Here's how the part is built. I have some questions about the finished solid (model axes, mm). A direction names the side the tool comes from. Round coordinates to 2 decimals unless told otherwise and drop trailing zeros. Write each loop counter-clockwise with the first axis right and the second up, starting at its lowest first coordinate (ties: lowest second). Pieces come first, ordered by that corner, then holes. Notation, with made-up numbers: (-38, -22.75) -> (0, -22.75) arc R20 cw to (0, -11.75) -> close; hole circle Ø8 at (45.5, 75.5). An arc over 180 degrees is marked (long way). Answer in a Markdown table with one row per item. Add a question column.
from build123d import *

# Parameters (mm, degrees)
BASE_EXTRUSION_DEPTH = 6
ESQUISSE2_W          = 2
ESQUISSE2_H          = 4.614800239
BOSS_EXTRU_1_DEPTH   = 1


with BuildPart() as part:
    # Esquisse1 → Base-Extrusion (new body)
    with BuildSketch(Plane.XY):
        with BuildLine():
            Line((-1.429070273, 4.791425482), (-1.172025132, 4.085199761))
            ThreePointArc((-1.172025132, 4.085199761), (0, 4.25), (1.172025132, 4.085199761))
            Line((1.172025132, 4.085199761), (1.429070273, 4.791425482))
            ThreePointArc((1.429070273, 4.791425482), (0, 5), (-1.429070273, 4.791425482))
        make_face()
    extrude(amount=BASE_EXTRUSION_DEPTH)

    # Esquisse2 → Boss.-Extru.1 (add)
    with BuildSketch(Plane.XY.offset(6)):
        with Locations((0, 6.69259988)):
            Rectangle(ESQUISSE2_W, ESQUISSE2_H)
    extrude(amount=BOSS_EXTRU_1_DEPTH)


solid = part.part
Item 1: For P1, Ø1.1, axis at y = 5.5, z = 6.5, coming from the -X side; P2, Ø0.5, axis at y = 7, z = 6.5, coming from the +X side; P3, Ø1.6, axis at x = -0.5, y = 7.5, coming from the -Z side, each with a flat end and sliding along its axis, tell me the tip position at first contact or that it passes through.
Item 2: If we section it at B-B on x = 0.55: Please give me the cut outline in (y, z).
Item 3: I need wall thicknesses on line 1 along X through (y, z) = (5.45, 6.5); line 2 along Z through (x, y) = (0.5, 5.5); line 3 along Y through (x, z) = (0.05, 6.25). Which ranges of each line are inside material? Lowest first, please. Write a range as from..to.
Item 4: If we section it at C-C on z = 6.75: Please give me the cut outline in (x, y), then the cut area to 3 significant figures.
Item 5: If we mould it in two halves opening along X, with no side actions, what happens to faces 1 (the flat face through (1, 6.7, 6.5)), 2 (the flat face through (0, 4.385, 6.5)), 3 (the cylindrical face through (-0.02, 4.25, 2.96))? For each: pulls with the +X half, pulls with the -X half, needs draft (parallel to the pull), parting line crosses it, or undercut.
Item 6: If we section it at D-D on x = -0.15: Please give me the cut outline in (y, z), then the cut area to 3 significant figures.
Item 7: If we section it at A-A on y = 6.65: Please give me the cut outline in (x, z), then the cut area to 3 significant figures.
Item 8: On a 3-axis mill with a long thin cutter (end or side, diameter ignored), from which of +Z, -Z, +X, -X, +Y, -Y can I reach the whole of each face in a straight line? I mean faces 4 (the flat face through (0, 7, 7)), 5 (the cylindrical face through (0, 5, 3)). Say none if no direction works.
Results list:
| question | item | result |
|---|---|---|
| 1 | P1 | x = -1 |
| 1 | P2 | x = 1 |
| 1 | P3 | z = 6 |
| 2 | outline | (4.21, 0) -> (4.97, 0) -> (4.97, 6) -> (9, 6) -> (9, 7) -> (4.39, 7) -> (4.39, 6) -> (4.21, 6) -> close |
| 3 | line 1 | -1..1 |
| 3 | line 2 | 6..7 |
| 3 | line 3 | 4.39..9 |
| 4 | outline | (-1, 4.39) -> (1, 4.39) -> (1, 9) -> (-1, 9) -> close |
| 4 | area | 9.23 mm² |
| 5 | face 1 | pulls with the +X half |
| 5 | face 2 | needs draft |
| 5 | face 3 | undercut |
| 6 | outline | (4.25, 0) -> (5, 0) -> (5, 6) -> (9, 6) -> (9, 7) -> (4.39, 7) -> (4.39, 6) -> (4.25, 6) -> close |
| 6 | area | 9.12 mm² |
| 7 | outline | (-1, 6) -> (1, 6) -> (1, 7) -> (-1, 7) -> close |
| 7 | area | 2.00 mm² |
| 8 | face 4 | +Z, +X, -X, +Y, -Y |
| 8 | face 5 | -Z, +Y |
